Geometry: final body of the model. Coordinates: model frame, mm. Face numbers are marked on the shaded views. A direction names the side the tool comes from. Give positions to 0.01 mm unless a question says otherwise; leave off trailing zeros. Write each loop counter-clockwise with the first axis right and the second up, starting at its lowest first coordinate (ties: lowest second). Pieces come first, ordered by that corner, then holes. Notation, with made-up numbers: (-17, 65.5) - (2, 65.5) arc R32 cw to (2, 91.5) - close; hole circle Ø11 at (53.25, 57.25). An arc over 180 degrees is marked (long way). Return JSON: item names as keys, results as strings.
from build123d import *

# Parameters (mm, degrees)
F0_R          = 9
F0_R_2        = 5
F1_DEPTH      = 14
F1_DEPTH_BACK = 14
F0_R_3        = 9.5
F2_DEPTH      = 14.5
F2_DEPTH_BACK = 14.5


with BuildPart() as f1:
    # F0 (on Front) → F1 (new body, two sides)
    with BuildSketch(Plane.XZ) as f1_sk:
        Circle(F0_R)
        Circle(F0_R_2, mode=Mode.SUBTRACT)
    extrude(amount=F1_DEPTH)
    extrude(f1_sk.sketch, amount=-F1_DEPTH_BACK)

    # F0 (on Front) → F2 (join, two sides)
    with BuildSketch(Plane.XZ) as f2_sk:
        Circle(F0_R_3)
        Circle(F0_R, mode=Mode.SUBTRACT)
    extrude(amount=F2_DEPTH)
    extrude(f2_sk.sketch, amount=-F2_DEPTH_BACK)


solid = f1.part
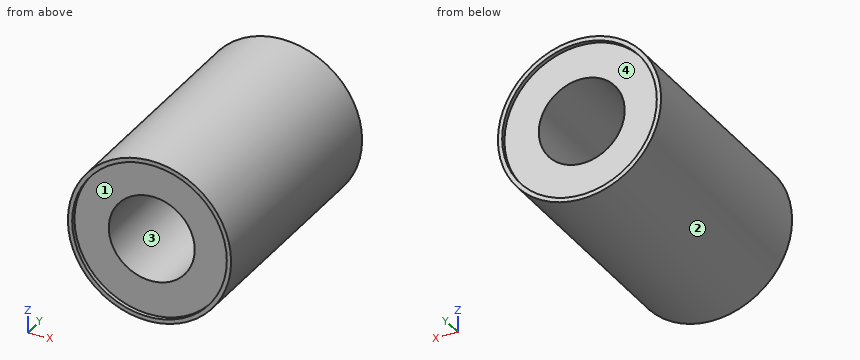
Q1. Mould query, pull axis X, two halves, no side actions, for the marked faces 1 and 2. Classes: pulls with the +X half, pulls with the -X half, needs draft (parallel to the pull), parting line crosses it, or undercut.
Answer key:
{"face 1": "undercut", "face 2": "parting line crosses it"}
Q2. Set-up query: the marked faces 3 and 4. Return all of +Z, -Z, +X, -X, +Y, -Y with unobstructed straight access to the full face (end or side cutting, diameter ignored); none if empty.
Answer key:
{"face 3": "+Y, -Y", "face 4": "+Y"}
Q3. Section query D-D, the plane x = 8.5. Return the cut outline in (y, z).
Answer key:
{"outline": "(-14.5, -4.24) - (14.5, -4.24) - (14.5, -2.96) - (14, -2.96) - (14, 2.96) - (14.5, 2.96) - (14.5, 4.24) - (-14.5, 4.24) - (-14.5, 2.96) - (-14, 2.96) - (-14, -2.96) - (-14.5, -2.96) - close"}
Q4. Section query B-B, the plane z = 0. Return the cut outline in (x, y).
Answer key:
{"outline": "(-9.5, -14.5) - (-9, -14.5) - (-9, -14) - (-5, -14) - (-5, 14) - (-9, 14) - (-9, 14.5) - (-9.5, 14.5) - close; (5, -14) - (9, -14) - (9, -14.5) - (9.5, -14.5) - (9.5, 14.5) - (9, 14.5) - (9, 14) - (5, 14) - close"}
Q5. Section query A-A, the plane x = 0. Return the cut outline in (y, z), plus the area to 3 significant figures.
Answer key:
{"outline": "(-14.5, -9.5) - (14.5, -9.5) - (14.5, -9) - (14, -9) - (14, -5) - (-14, -5) - (-14, -9) - (-14.5, -9) - close; (-14.5, 9) - (-14, 9) - (-14, 5) - (14, 5) - (14, 9) - (14.5, 9) - (14.5, 9.5) - (-14.5, 9.5) - close", "area": "253 mm^2"}
Q6. Pin query (flat end, axial travel): P1, Ø1.5, axis at y = 8, z = -6, coming from the +X side; P2, Ø3, axis at y = -4.5, z = -4.5, coming from the -X side; P3, Ø6, axis at y = -4, z = -6.5, coming from the -X side. Return the tip coordinate at first contact, or that it passes through.
Answer key:
{"P1": "stops at x = 7.92", "P2": "stops at x = -9.01", "P3": "stops at x = -8.83"}
Q7. Material intervals for probe 1 along Z at (x, y) = (0, 4); probe 2 along Z at (x, y) = (0, 14.35); probe 3 along Y at (x, z) = (2.5, -5), sorted ascending. Write a range as [from, to].
Answer key:
{"probe 1": "z = [-9.5, -5], [5, 9.5]", "probe 2": "z = [-9.5, -9], [9, 9.5]", "probe 3": "y = [-14, 14]"}
Q8. Section query C-C, the plane y = -12.5. Return the cut outline in (x, z).
Answer key:
{"outline": "circle Ø19 at (0, 0); hole circle Ø10 at (0, 0)"}
